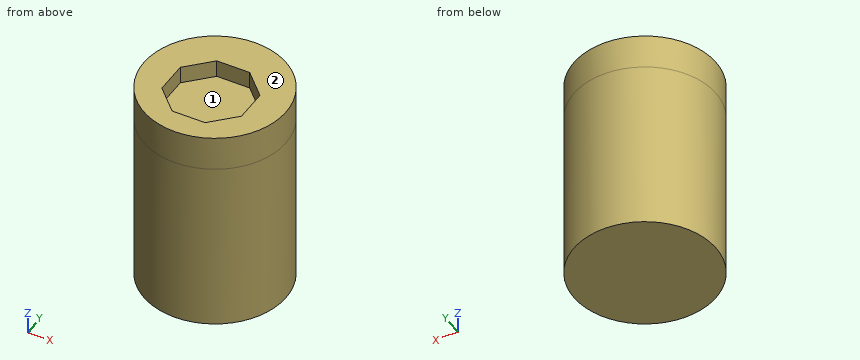
```python
from build123d import *

# Parameters (mm, degrees)
F0_R     = 51.8043549738
F1_DEPTH = 76.2
F2_DEPTH = 25.4
F3_DEPTH = 25.4
F5_DEPTH = 12.7
F6_DEPTH = 127


with BuildPart() as f1:
    # F0 (on Top) → F1 (new body)
    with BuildSketch(Plane.XY):
        Circle(F0_R)
    extrude(amount=F1_DEPTH)

    # F2 (cut): a face of the model
    f2_faces = [f1.faces().sort_by_distance(p)[0] for p in [
        (0, 0, 76.2),
    ]]
    extrude(f2_faces, amount=-F2_DEPTH, mode=Mode.SUBTRACT)

    # F3 (cut): a face of the model
    f3_faces = [f1.faces().sort_by_distance(p)[0] for p in [
        (0, 0, 50.8),
    ]]
    extrude(f3_faces, amount=-F3_DEPTH, mode=Mode.SUBTRACT)

    # F4 (on face) → F5 (cut)
    with BuildSketch(Plane.XY.offset(25.4)):
        Polygon((29.0936566889, -17.3791157596), (29.0936566889, 6.7228585996), (12.0509871796, 23.7655281089), (-12.0509871796, 23.7655281089), (-29.0936566889, 6.7228585996), (-29.0936566889, -17.3791157596), (-12.0509871796, -34.4217852689), (12.0509871796, -34.4217852689), align=None)
    extrude(amount=-F5_DEPTH, mode=Mode.SUBTRACT)

    # F6 (add): a face of the model
    f6_faces = [f1.faces().sort_by_distance(p)[0] for p in [
        (0, 0, 0),
    ]]
    extrude(f6_faces, amount=F6_DEPTH)


solid = f1.part
```
The listing builds one solid part. Answer for the finished solid, in the listing's coordinates (mm). Face numbers are marked on the shaded views. Give positions to 0.01 mm unless a question says otherwise; leave off trailing zeros. Order: outer loops, then holes, each group sorted by start corner. A loop starts at its lowest first (then second) coordinate and runs counter-clockwise, first axis right, second up. Notation, with made-up numbers: (0.5, 41.25) - (47.5, 41.25) arc R18 cw to (47.5, 60.25) - close; hole circle Ø1 at (-32.5, 50). An arc over 180 degrees is marked (long way). Answer in a Markdown table with one row per item. Add a question column.
Q1. The part is cut by section C-C (z = -99). Determine the outline of the cut face in (x, y).
Q2. The part is cut by section D-D (y = 39). Determine the outline of the cut face in (x, z), then the cut area to 3 significant figures.
Q3. Given P1, Ø5, axis at y = 40, z = -80, coming from the +X side; P2, Ø3, axis at x = 6, y = -27, coming from the +Z side; P3, Ø2, axis at y = 11.5, z = -44, coming from the -X side, each flat-ended and moving along its own axis, determine where each tip first touches the part or whether it passes through.
Q4. The part is cut by section B-B (y = 0). Determine the outline of the cut face in (x, z).
Q5. Find the intervals of material crossed by line 1 along Z through (x, y) = (-6, -17); line 2 along Y through (x, z) = (-18.5, 15.5); line 3 along Y through (x, z) = (14.5, -74.5), in increasing order. Write a range as [from, to].
Q6. The part is cut by section A-A (x = 0). Determine the outline of the cut face in (y, z), then the cut area to 3 significant figures.
Q7. For a pull along X with two mould halves and no side action, classify the marked faces 1 and 2 as released by +X, released by -X, zero draft, split by the parting line, or undercut.
Determined:
| question | item | result |
|---|---|---|
| 1 | outline | circle Ø103.61 at (0, 0) |
| 2 | outline | (-34.1, -127) - (34.1, -127) - (34.1, 25.4) - (-34.1, 25.4) - close |
| 2 | area | 10,400 mm² |
| 3 | P1 | stops at x = 35.74 |
| 3 | P2 | stops at z = 12.7 |
| 3 | P3 | stops at x = -50.73 |
| 4 | outline | (-51.8, -127) - (51.8, -127) - (51.8, 25.4) - (29.09, 25.4) - (29.09, 12.7) - (-29.09, 12.7) - (-29.09, 25.4) - (-51.8, 25.4) - close |
| 5 | line 1 | z = [-127, 12.7] |
| 5 | line 2 | y = [-48.39, -27.97], [17.32, 48.39] |
| 5 | line 3 | y = [-49.73, 49.73] |
| 6 | outline | (-51.8, -127) - (51.8, -127) - (51.8, 25.4) - (23.77, 25.4) - (23.77, 12.7) - (-34.42, 12.7) - (-34.42, 25.4) - (-51.8, 25.4) - close |
| 6 | area | 15,100 mm² |
| 7 | face 1 | undercut |
| 7 | face 2 | zero draft |
